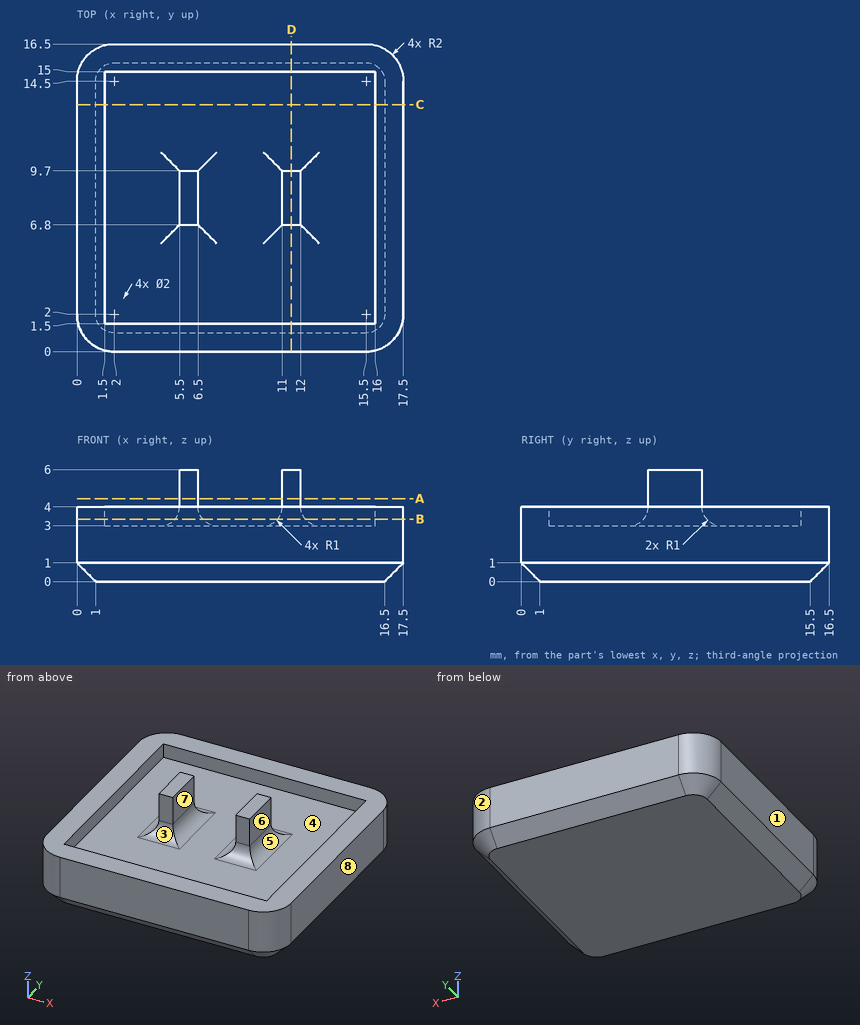
For this review, use the dimensioned drawing (mm, ordinates from the lowest corner) and the shaded views. A direction names the side the tool comes from. Round coordinates to 2 decimals unless told otherwise and drop trailing zeros. Write each loop counter-clockwise with the first axis right and the second up, starting at its lowest first coordinate (ties: lowest second). Pieces come first, ordered by that corner, then holes. Notation, with made-up numbers: (-27.5, 24) - (7.5, 24) arc R19 ccw to (7.5, 45) - close; hole circle Ø5 at (80.25, 62). An arc over 180 degrees is marked (long way). One line per item, written item: value. Start each with the question number.
1. Consider section C-C on y = 13.25. Write out the cut boundary in (x, z), and give its area (3 significant figures).
2. Consider section B-B on z = 3.35. Write out the cut boundary in (x, y).
3. Machinability: for the marked faces 5, 6, 7 and 8, which of the approach directions +Z, -Z, +X, -X, +Y, -Y give a long, thin tool a straight path to every point of the face, cutting with its end or side? Answer none if there is none.
4. Clearance check with flat-ended pins moving along their axes: P1, Ø3, axis at y = 13, z = 3.5, coming from the -X side; P2, Ø0.6, axis at y = 9, z = 5.5, coming from the +X side; P3, Ø0.5, axis at x = 6, z = 4.5, coming from the -Y side; P4, Ø1.6, axis at y = 8.5, z = 5, coming from the -X side. State where each tip first meets the part, or that it passes through.
5. To check wall thickness, follow L1, parallel to X at y = 7.5, z = 4.2; L2, parallel to Y at x = 4, z = 3.35; L3, parallel to X at y = 14.5, z = 3.05. State the ranges of each line that lie inside material, in increasing order. Write a range as from..to.
6. Consider section A-A on z = 4.45. Write out the cut boundary in (x, y), and give its area (3 significant figures).
7. Consider section D-D on x = 11.5. Write out the cut boundary in (y, z), and give its area (3 significant figures).
8. The part is to be moulded in two halves that separate along Y. For the marked faces 1, 2, 3 and 4, say which applies: released by +Y, released by -Y, zero draft, split by the parting line, or undercut.
Checks:
1. outline: (0, 1) - (1, 0) - (16.5, 0) - (17.5, 1) - (17.5, 4) - (16, 4) - (16, 3) - (1.5, 3) - (1.5, 4) - (0, 4) - close
1. area: 54.5 mm^2
2. outline: (0, 2) arc R2 ccw to (2, 0) - (15.5, 0) arc R2 ccw to (17.5, 2) - (17.5, 14.5) arc R2 ccw to (15.5, 16.5) - (2, 16.5) arc R2 ccw to (0, 14.5) - close; (5.26, 6.56) - (6.74, 6.56) - (6.74, 9.94) - (5.26, 9.94) - close; (10.76, 6.56) - (12.24, 6.56) - (12.24, 9.94) - (10.76, 9.94) - close; hole (1.5, 1.5) - (16, 1.5) - (16, 15) - (1.5, 15) - close
3. face 5: +Z
3. face 6: +Z, +X, +Y, -Y
3. face 7: +Z, +Y, -Y
3. face 8: +Z, -Z, +X, +Y, -Y
4. P1: stops at x = 0
4. P2: stops at x = 12
4. P3: stops at y = 6.8
4. P4: stops at x = 5.5
5. L1: x = 5.5..6.5, 11..12
5. L2: y = 0..1.5, 15..16.5
5. L3: x = 0..1.5, 16..17.5
6. outline: (5.5, 6.8) - (6.5, 6.8) - (6.5, 9.7) - (5.5, 9.7) - close; (11, 6.8) - (12, 6.8) - (12, 9.7) - (11, 9.7) - close
6. area: 5.80 mm^2
7. outline: (0, 1) - (1, 0) - (15.5, 0) - (16.5, 1) - (16.5, 4) - (15, 4) - (15, 3) - (10.7, 3) arc R1 cw to (9.7, 4) - (9.7, 6) - (6.8, 6) - (6.8, 4) arc R1 cw to (5.8, 3) - (1.5, 3) - (1.5, 4) - (0, 4) - close
7. area: 60.6 mm^2
8. face 1: zero draft
8. face 2: released by +Y
8. face 3: undercut
8. face 4: undercut
